Source: CAD feature listing. Evaluate the final solid. Frame: model axes, mm. Face numbers are marked on the shaded views. A direction names the side the tool comes from. Give positions to 0.01 mm unless a question says otherwise; leave off trailing zeros. Write each loop counter-clockwise with the first axis right and the second up, starting at its lowest first coordinate (ties: lowest second). Pieces come first, ordered by that corner, then holes. Notation, with made-up numbers: (-4.5, -4.5) -> (8.5, -4.5) arc R24 cw to (8.5, 28.5) -> close; hole circle Ø6 at (4, 77.25). An arc over 180 degrees is marked (long way). Write item = value, one per line.
Autodesk Fusion 360 part; units mm, degrees
sketch "Esboço1" plane through (0, 0, 0) normal (0, 1, 0) x (1, 0, 0)
  line L0 (0, 0) -> (95, 0)
  line L1 (95, 0) -> (95, -93)
  line L2 (95, -93) -> (0, -93)
  line L3 (0, -93) -> (0, 0)
  dimension "d1" = 95
  dimension "d2" = 93
extrude "Extrusão1" add sketch "Esboço1" along normal blind 15
sketch "Esboço2" plane through (0, 15, 0) normal (0, 1, 0) x (-1, 0, 0)
  line L0 (0, 93) -> (-95, 93)
  line L1 (-95, 93) -> (-95, 0)
  line L2 (-95, 0) -> (0, 0)
  line L3 (0, 0) -> (0, 93)
  line L4 (-94, 91) -> (-50, 91)
  line L5 (-50, 91) -> (-50, 9)
  line L6 (-50, 9) -> (-94, 9)
  line L7 (-94, 9) -> (-94, 91)
  line L8 (-45, 91) -> (-1, 91)
  line L9 (-1, 91) -> (-1, 9)
  line L10 (-1, 9) -> (-45, 9)
  line L11 (-45, 9) -> (-45, 91)
  dimension "d10" = 44
  dimension "d11" = 82
  dimension "d12" = 44
  dimension "d13" = 82
  dimension "d14" = 1
  dimension "d15" = 1
  dimension "d16" = 5
extrude "Extrusão2" cut sketch "Esboço2" against normal blind 5.5 contours L4 L5 L6 L7 | L8 L9 L10 L11
fillet "Arredondamento2" radius 5.499 8 edges at (94, 9.5, 50) (72, 9.5, 91) (50, 9.5, 50) (72, 9.5, 9) (50, 12.25, 91) (94, 12.25, 91) (94, 12.25, 9) (50, 12.25, 9)
fillet "Arredondamento3" radius 5.4999 8 edges at (45, 9.5, 50) (23, 9.5, 9) (45, 12.25, 9) (45, 12.25, 91) (23, 9.5, 91) (1, 12.25, 91) (1, 9.5, 50) (1, 12.25, 9)
sketch "Esboço3" plane through (0, 9.5, 0) normal (0, 1, 0) x (-1, 0, 0)
  line L0 (-55.499, 14.499) -> (-55.499, 85.501)
  line L1 (-55.499, 85.501) -> (-88.501, 85.501)
  line L2 (-88.501, 85.501) -> (-88.501, 14.499)
  line L3 (-88.501, 14.499) -> (-55.499, 14.499)
  line L4 (-88.501, 14.499) -> (-93.501, 9.499)
  line L5 (-88.501, 14.499) -> (-80.8219, 14.499) construction
  line L6 (-93.501, 9.499) -> (-88.501, 9.499)
  line L7 (-88.501, 14.499) -> (-93.501, 14.499)
  line L8 (-93.501, 14.499) -> (-95, 14.499)
  line L9 (-89.7081, 13.999) -> (-93.8546, 9.8526)
  line L10 (-89.7081, 13.999) -> (-93.501, 13.999)
  line L11 (-93.501, 13.999) -> (-95, 13.999)
  line L12 (-93.501, 9.199) -> (-88.501, 9.199)
  line L13 (-93.8546, 9.8526) -> (-94.5081, 9.199)
  line L14 (-94.5081, 9.199) -> (-93.501, 9.199)
  dimension "d21" = 135
  dimension "d22" = 5
  dimension "d23" = -0.5
  dimension "d24" = 0.3
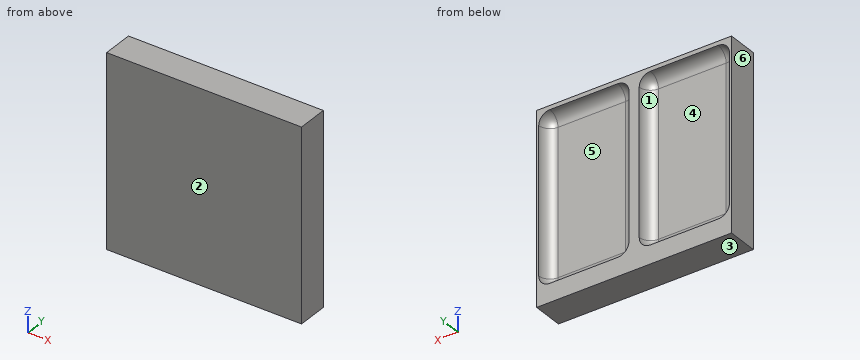
(1) First-contact query: pin 1 (6 mm diameter, centred on x = 20, z = 54.5, fed in from +Y). Flat tip, straight axial feed; report the tip coordinate or a pass-through.
Values follow:
pin_1 = 9.5
(2) Pull-direction query (Z, two-part tool) for the marked faces 3, 4, 5 and 6; classes: pulls with the +Z half, pulls with the -Z half, needs draft (parallel to the pull), parting line crosses it, or undercut.
Values follow:
face_3 = pulls with the -Z half
face_4 = undercut
face_5 = undercut
face_6 = needs draft
(3) Material intervals for line 1 (X direction, y = 14.25, z = 87); line 2 (X direction, y = 13, z = 65.5); line 3 (Y direction, x = 57.5, z = 29.5), sorted ascending.
Values follow:
line_1 = 0 to 1.26, 44.74 to 50.26, 93.74 to 95
line_2 = 0 to 1.38, 44.62 to 50.38, 93.62 to 95
line_3 = 0 to 9.5
(4) Section query B-B (y = 11). Return loops of the section in (x, z), plus the area to 3 significant figures.
Values follow:
outline = (0, 0) -> (95, 0) -> (95, 93) -> (0, 93) -> close; hole (2.73, 14.5) arc R3.77 ccw to (6.5, 10.73) -> (39.5, 10.73) arc R3.77 ccw to (43.27, 14.5) -> (43.27, 85.5) arc R3.77 ccw to (39.5, 89.27) -> (6.5, 89.27) arc R3.77 ccw to (2.73, 85.5) -> close; hole (51.72, 14.5) arc R3.77 ccw to (55.5, 10.72) -> (88.5, 10.72) arc R3.77 ccw to (92.28, 14.5) -> (92.28, 85.5) arc R3.77 ccw to (88.5, 89.28) -> (55.5, 89.28) arc R3.77 ccw to (51.72, 85.5) -> close
area = 2,490 mm2
(5) Access query for the marked faces 1 and 2. Directions: +Z, -Z, +X, -X, +Y, -Y. A direction counts if a zero-diameter tool reaches every point of the face in a straight line with its end or side. Return the directions, or none.
Values follow:
face_1 = +Y
face_2 = +Z, -Z, +X, -X, -Y
